Geometry check sheet. Reference: the model listing, model coordinates, mm. A direction names the side the tool comes from. Round coordinates to 2 decimals unless told otherwise and drop trailing zeros. Loops run counter-clockwise (first coordinate to the right, second up) from the corner with the lowest first, then second, coordinate; pieces in that order, holes last. Notation, with made-up numbers: M 80.25,51 L 136.25,51 A12 ccw 136.25,68 Z; hole C 71.5,54.25 d9. An arc over 180 degrees is marked long. Answer in a Markdown table with one row per item. Add a question column.
```python
from build123d import *

# Parameters (mm, degrees)
SKETCH1_R             = 22.4
EXTRUDE1_DEPTH        = 70
SKETCH2_R             = 16.15
EXTRUDE2_DEPTH        = 64
SKETCH3_R             = 5
EXTRUDE3_DEPTH        = 10
EXTRUDE5_DEPTH        = 30
M5_TAPPED_HOLE3_D     = 4.2
M5_TAPPED_HOLE5_D     = 4.2
M5_TAPPED_HOLE5_DEPTH = 14
M5_TAPPED_HOLE5_TIP   = 1.2618073
M4_TAPPED_HOLE1_D     = 3.3
M4_TAPPED_HOLE1_DEPTH = 11.5
M4_TAPPED_HOLE1_TIP   = 0.991420021


with BuildPart() as part:
    # Sketch1 → Extrude1 (new body)
    with BuildSketch(Plane(origin=(0, 0, 0), x_dir=(0, 0, -1), z_dir=(1, 0, 0))):
        Circle(SKETCH1_R)
    extrude(amount=EXTRUDE1_DEPTH)

    # Sketch2 → Extrude2 (cut)
    with BuildSketch(Plane(origin=(70, 0, 0), x_dir=(0, 0, -1), z_dir=(1, 0, 0))):
        Circle(SKETCH2_R)
    extrude(amount=-EXTRUDE2_DEPTH, mode=Mode.SUBTRACT)

    # Sketch3 → Extrude3 (cut)
    with BuildSketch(Plane.ZY):
        Circle(SKETCH3_R)
    extrude(amount=-EXTRUDE3_DEPTH, mode=Mode.SUBTRACT)

    # Sketch7 → Extrude5 (cut)
    with BuildSketch(Plane(origin=(0, 0, 0), x_dir=(1, 0, 0), z_dir=(0, 1, 0))):
        with BuildLine():
            Line((9, 12.5), (43, 12.5))
            ThreePointArc((43, 12.5), (45.121320344, 11.621320344), (46, 9.5))
            Line((46, 9.5), (46, -9.5))
            ThreePointArc((46, -9.5), (45.121320344, -11.621320344), (43, -12.5))
            Line((43, -12.5), (9, -12.5))
            ThreePointArc((9, -12.5), (6.878679656, -11.621320344), (6, -9.5))
            Line((6, -9.5), (6, 9.5))
            ThreePointArc((6, 9.5), (6.878679656, 11.621320344), (9, 12.5))
        make_face()
    extrude(amount=-EXTRUDE5_DEPTH, mode=Mode.SUBTRACT)

    # M5 Tapped Hole3 (through all)
    with Locations(Plane(origin=(60, 0, 22.4), x_dir=(1, 0, 0), z_dir=(0, 0, 1))):
        with Locations((0, 0)):
            Hole(M5_TAPPED_HOLE3_D / 2)

    # M5 Tapped Hole5
    with Locations(Plane(origin=(59.947350676, -16.149783021, -0.083715942), x_dir=(0, -0.005183649651, 0.999986564798), z_dir=(0, 0.999986564798, 0.005183649651))):
        with Locations((0, 0)):
            Hole(M5_TAPPED_HOLE5_D / 2, depth=M5_TAPPED_HOLE5_DEPTH)
            with Locations((0, 0, -(M5_TAPPED_HOLE5_DEPTH + M5_TAPPED_HOLE5_TIP / 2))):  # 118° drill point
                Cone(0, M5_TAPPED_HOLE5_D / 2, M5_TAPPED_HOLE5_TIP, mode=Mode.SUBTRACT)

    # M4 Tapped Hole1
    with Locations(Plane(origin=(0, 0, -15.027388536), x_dir=(0, 0, -1), z_dir=(-1, 0, 0))):
        with Locations((0, 0), (-15.027388536, -15), (-30.027388536, 0), (-15.027388536, 15)):
            Hole(M4_TAPPED_HOLE1_D / 2, depth=M4_TAPPED_HOLE1_DEPTH)
            with Locations((0, 0, -(M4_TAPPED_HOLE1_DEPTH + M4_TAPPED_HOLE1_TIP / 2))):  # 118° drill point
                Cone(0, M4_TAPPED_HOLE1_D / 2, M4_TAPPED_HOLE1_TIP, mode=Mode.SUBTRACT)


solid = part.part
```
1) Go/stop test with flat-tipped pins: pin 1 (2 mm diameter, centred on x = 32.5, y = 3, fed in from -Z); pin 2 (12 mm diameter, centred on x = 11, y = 9.5, fed in from +Z); pin 3 (6.5 mm diameter, centred on x = 20, y = -16, fed in from +Z). Record where each tip stops, or that it passes through.
2) Thickness scan on L1, parallel to Y at x = 4, z = 0; L2, parallel to Y at x = 2.5, z = 15. Record the ranges inside material, lowest first. Write a range as [from, to].
3) Draft check along Y on faces 6 (the cylindrical face through (4.6, 16.6, -0.4)), 7 (the cylindrical face through (34.51, 22.21, 2.92)), 8 (the cylindrical face through (45.1, -15.19, -11.64)). Enter one of: +Y half, -Y half, draft (parallel to the pull), parting line (faces both ways), or undercut.
4) Cross-section at A-A, the plane y = 0. Record the boundary of the cut face in (x, z), plus the area to 3 significant figures.
5) Cross-section at D-D, the plane x = 65.5. Record the boundary of the cut face in (y, z), plus the area to 3 significant figures.
6) Cross-section at C-C, the plane y = 15. Record the boundary of the cut face in (x, z), plus the area to 3 significant figures.
7) Cross-section at B-B, the plane z = 10.5. Record the boundary of the cut face in (x, y), plus the area to 3 significant figures.
8) Set-up check for faces 1 (the flat face through (6, -7, 0)), 2 (the flat face through (0, 5.3, 0.3)), 3 (the cylindrical face through (38.448, 16.013, 2.102)), 4 (the cylindrical face through (3.04, -16.39, 0.89)), 5 (the cylindrical face through (6.9, -15.19, 11.64)): record each of +Z, -Z, +X, -X, +Y, -Y from which the full face is reachable in a straight line by a thin tool's end or side.
Worked answers:
| question | item | result |
|---|---|---|
| 1 | pin 1 | stops at z = -22.31 |
| 1 | pin 2 | stops at z = 22.12 |
| 1 | pin 3 | stops at z = 18.42 |
| 2 | L1 | y = [-22.4, -16.65], [-13.35, -5], [5, 13.35], [16.65, 22.4] |
| 2 | L2 | y = [-16.64, -1.65], [1.65, 16.64] |
| 3 | face 6 | undercut |
| 3 | face 7 | parting line |
| 3 | face 8 | draft |
| 4 | outline | M 0,-22.4 L 57.9,-22.4 L 57.9,-16.15 L 11.82,-16.15 L 11.5,-16.68 L 0,-16.68 Z; M 0,-13.38 L 6,-13.38 L 6,-5 L 0,-5 Z; M 0,5 L 6,5 L 6,13.35 L 0,13.35 Z; M 0,16.65 L 11.5,16.65 L 11.8,16.15 L 57.9,16.15 L 57.9,22.4 L 0,22.4 Z; M 62.1,-22.4 L 70,-22.4 L 70,-16.15 L 62.1,-16.15 Z; M 62.1,16.15 L 70,16.15 L 70,22.4 L 62.1,22.4 Z |
| 4 | area | 911 mm2 |
| 5 | outline | C 0,0 d44.8; hole C 0,0 d32.3 |
| 5 | area | 757 mm2 |
| 6 | outline | M 0,-16.64 L 70,-16.64 L 70,-5.99 L 6,-5.99 L 6,-1.65 L 0,-1.65 Z; M 0,1.65 L 6,1.65 L 6,5.99 L 70,5.99 L 70,16.64 L 0,16.64 Z |
| 6 | area | 1,540 mm2 |
| 7 | outline | M 0,-19.79 L 6.17,-19.79 L 6.17,-12.27 L 6,-12.27 L 6,12.27 L 70,12.27 L 70,19.79 L 0,19.79 Z; M 45.83,-19.79 L 70,-19.79 L 70,-12.27 L 45.83,-12.27 Z |
| 7 | area | 901 mm2 |
| 8 | face 1 | none |
| 8 | face 2 | +Z, -Z, -X, +Y, -Y |
| 8 | face 3 | +X |
| 8 | face 4 | -X |
| 8 | face 5 | -Y |
